Read the model definition and answer for the solid it produces. Units are mm, in the model's axes. Coordinates: 2 decimals unless noted, no trailing zeros. Write each loop counter-clockwise with the first axis right and the second up, starting at its lowest first coordinate (ties: lowest second). Pieces come first, ordered by that corner, then holes. Notation, with made-up numbers: (79, 58) -> (130, 58) arc R17 ccw to (130, 70) -> close; hole circle Ø6 at (-7, 25.25). An arc over 180 degrees is marked (long way). Return JSON: item names as keys, results as strings.
from build123d import *

# Parameters (mm, degrees)
F0_W     = 100
F0_H     = 50
F0_R     = 2
F0_R_2   = 15
F1_DEPTH = 3
F2_R     = 20


with BuildPart() as f1:
    # F0 (on Front) → F1 (new body)
    with BuildSketch(Plane.XZ):
        Rectangle(F0_W, F0_H)
        with Locations((-36, 10)):
            Circle(F0_R, mode=Mode.SUBTRACT)
        Circle(F0_R_2, mode=Mode.SUBTRACT)
        with Locations((36, 10)):
            Circle(F0_R, mode=Mode.SUBTRACT)
    extrude(amount=F1_DEPTH)

    # F2
    f2_edges = [f1.edges().sort_by_distance(p)[0] for p in [
        (-50, -1.5, 25),
        (50, -1.5, 25),
    ]]
    fillet(f2_edges, radius=F2_R)


solid = f1.part
1. The part is cut by section D-D (z = 10). Determine the outline of the cut face in (x, y).
Taken from the geometry:
{"outline": "(-49.36, -3) -> (-38, -3) -> (-38, 0) -> (-49.36, 0) -> close; (-34, -3) -> (-11.18, -3) -> (-11.18, 0) -> (-34, 0) -> close; (11.18, -3) -> (34, -3) -> (34, 0) -> (11.18, 0) -> close; (38, -3) -> (49.36, -3) -> (49.36, 0) -> (38, 0) -> close"}
2. The part is cut by section A-A (z = 0). Determine the outline of the cut face in (x, y).
Taken from the geometry:
{"outline": "(-50, -3) -> (-15, -3) -> (-15, 0) -> (-50, 0) -> close; (15, -3) -> (50, -3) -> (50, 0) -> (15, 0) -> close"}
3. Flat-ended cylindrical pins translate along their axes: pin 1 Ø1 at (y, z) = (-1.5, 19.5) entering from -X; pin 2 Ø1 at (x, z) = (28, 15.5) entering from +Y. Find the tip coordinate at first contact, or state that the pin passes through.
Taken from the geometry:
{"pin 1": "stops at x = -44.28", "pin 2": "stops at y = 0"}
4. The part is cut by section C-C (x = -12.5). Determine the outline of the cut face in (y, z).
Taken from the geometry:
{"outline": "(-3, -25) -> (0, -25) -> (0, -8.29) -> (-3, -8.29) -> close; (-3, 8.29) -> (0, 8.29) -> (0, 25) -> (-3, 25) -> close"}
5. The part is cut by section B-B (y = -2.45). Determine the outline of the cut face in (x, z), then the cut area to 3 significant figures.
Taken from the geometry:
{"outline": "(-50, -25) -> (50, -25) -> (50, 5) arc R20 ccw to (30, 25) -> (-30, 25) arc R20 ccw to (-50, 5) -> close; hole circle Ø4 at (-36, 10); hole circle Ø30 at (0, 0); hole circle Ø4 at (36, 10)", "area": "4,100 mm2"}
6. Consider L1, parallel to Z at x = 0, y = -1.1; L2, parallel to Z at x = -4.5, y = -1.8; L3, parallel to Z at x = -30.5, y = -2.5. Determine where each line is inside the solid, lowest interval first.
Taken from the geometry:
{"L1": "z = -25 to -15, 15 to 25", "L2": "z = -25 to -14.31, 14.31 to 25", "L3": "z = -25 to 24.99"}
7. For a pull along X with two mould halves and no side action, classify faces 1 (the face through (-37.474, -1.479, 11.352)), 2 (the face through (-12, -3, -11)), 3 (the face through (-50, -1, -10)) as +X half, -X half, draft (parallel to the pull), parting line (faces both ways), or undercut.
Taken from the geometry:
{"face 1": "undercut", "face 2": "draft", "face 3": "-X half"}
